Source: CAD feature listing. Evaluate the final solid. Frame: model axes, mm. A direction names the side the tool comes from. Round coordinates to 2 decimals unless told otherwise and drop trailing zeros. Order: outer loops, then holes, each group sorted by start corner. A loop starts at its lowest first (then second) coordinate and runs counter-clockwise, first axis right, second up. Notation, with made-up numbers: M -13.75,27 L 0.25,27 A13 ccw 0.25,32 Z; hole C 65.5,85 d9. An arc over 180 degrees is marked long. Use one line per item in the form item = value. Start each with the question number.
Q1. Section A-A (y = -6.5). Return the cut outline in (x, z), plus the area to 3 significant figures.
Q2. Pull-direction query (Y, two-part tool) for faces 3 (the flat face through (-5.1, 5.2, -5.2)), 4 (the cylindrical face through (-2.514, 6.466, -2.681)), 5 (the cylindrical face through (-15.21, -1.341, 3.233)); classes: pulls with the +Y half, pulls with the -Y half, needs draft (parallel to the pull), parting line crosses it, or undercut.
Q3. Contact query for flat-ended pins moving along their axis: pin 1 (1.5 mm diameter, centred on y = -3.5, z = 8, fed in from -X); pin 2 (3 mm diameter, centred on x = -5.5, z = -4, fed in from +Y); pin 3 (10 mm diameter, centred on x = -20, z = -5.5, fed in from -Y). Output: stop coordinate, or through.
Q4. Material intervals for probe 1 along Z at (x, y) = (-13.25, 0); probe 2 along X at (y, z) = (-8.25, -2.5); probe 3 along Y at (x, z) = (-3, 2), sorted ascending.
Q5. Section B-B (z = -5.5). Return the cut outline in (x, y).
Q6. Section C-C (x = -44). Return the cut outline in (y, z), plus the area to 3 significant figures.
Q7. Reachability of faces 1 (the flat face through (0, 3, -3)), 2 (the flat face through (-12.1, -5.2, -5.2)) from +Z, -Z, +X, -X, +Y, -Y: full face, straight path, thin tool, end or side. Return the list, or none.
Q8. Section D-D (z = -9). Return the cut outline in (x, y).
from build123d import *

# Parameters (mm, degrees)
TROU_TARAUD_M8X1_01_D     = 7
TROU_TARAUD_M8X1_01_DEPTH = 30
TROU_TARAUD_M8X1_01_TIP   = 2.103012167


with BuildPart() as part:
    # Sketch1 → Revolve1 (revolve)
    with BuildSketch(Plane.XY):
        Polygon((-5.1, 12), (-5.1, 7), (0, 7), (0, 0), (-50, 0), (-50, 7), (-12.1, 7), (-12.1, 12), align=None)
    revolve(axis=Axis((-78.343949045, 0, 0), (1, 0, 0)))

    # Trou taraudé M8x1.01
    with Locations(Plane(origin=(0, 0, 0), x_dir=(0, 0, -1), z_dir=(1, 0, 0))):
        with Locations((0, 0)):
            Hole(TROU_TARAUD_M8X1_01_D / 2, depth=TROU_TARAUD_M8X1_01_DEPTH)
            with Locations((0, 0, -(TROU_TARAUD_M8X1_01_DEPTH + TROU_TARAUD_M8X1_01_TIP / 2))):  # 118° drill point
                Cone(0, TROU_TARAUD_M8X1_01_D / 2, TROU_TARAUD_M8X1_01_TIP, mode=Mode.SUBTRACT)


solid = part.part
Results list:
q1.outline = M -50,-2.6 L -12.1,-2.6 L -12.1,-10.09 L -5.1,-10.09 L -5.1,-2.6 L 0,-2.6 L 0,2.6 L -5.1,2.6 L -5.1,10.09 L -12.1,10.09 L -12.1,2.6 L -50,2.6 Z
q1.area = 365 mm2
q2.face_3 = needs draft
q2.face_4 = parting line crosses it
q2.face_5 = undercut
q3.pin_1 = -12.1
q3.pin_2 = 11.74
q3.pin_3 = -6.98
q4.probe_1 = -7 to -3.5, 3.5 to 7
q4.probe_2 = -12.1 to -5.1
q4.probe_3 = -6.71 to -2.87, 2.87 to 6.71
q5.outline = M -50,-4.33 L -12.1,-4.33 L -12.1,-10.67 L -5.1,-10.67 L -5.1,-4.33 L 0,-4.33 L 0,4.33 L -5.1,4.33 L -5.1,10.67 L -12.1,10.67 L -12.1,4.33 L -50,4.33 Z
q6.outline = C 0,0 d14
q6.area = 154 mm2
q7.face_1 = +Z, -Z, +X, +Y, -Y
q7.face_2 = -X
q8.outline = M -12.1,-7.94 L -5.1,-7.94 L -5.1,7.94 L -12.1,7.94 Z
